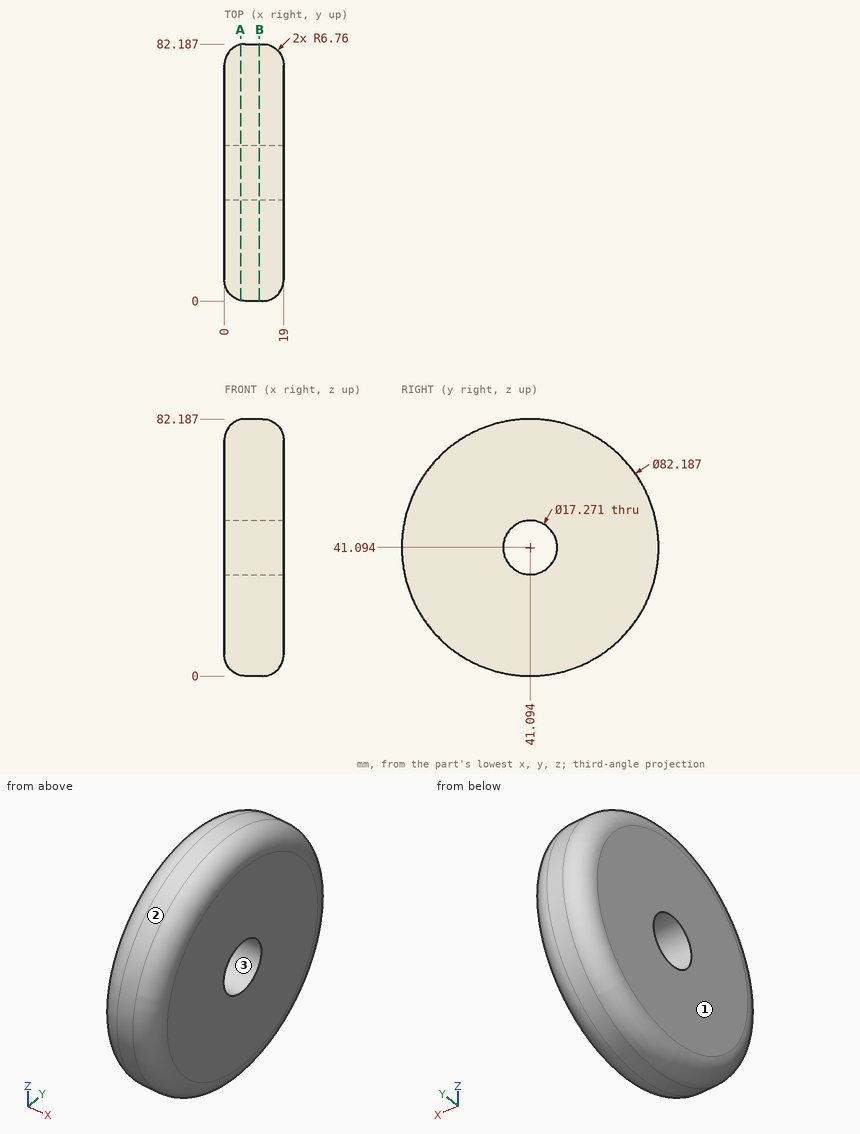
Geometry: see drawing. Coordinates: mm, zero at the bounding-box minimum. Coordinates: 2 decimals unless noted, no trailing zeros. Loops run counter-clockwise (first coordinate to the right, second up) from the corner with the lowest first, then second, coordinate; pieces in that order, holes last. Notation, with made-up numbers: M -1,58.25 L 45,58.25 A4 ccw 45,62.25 Z; hole C 2,-32.75 d3. An arc over 180 degrees is marked long. Put each result on its own line as item: value. Start each with the question number.
1) Cut plane A-A on x = 5.25. Return the cut outline in (y, z) (1 decimal), then the cut area to 3 significant figures.
2) Cut plane B-B on x = 11.25. Return the cut outline in (y, z) (1 decimal), then the cut area to 3 significant figures.
3) Ray query, L1, parallel to Z at x = 13.75, y = 39.5 (1 decimal); L2, parallel to Y at x = 7.75, z = 37.5 (1 decimal); L3, parallel to Z at x = 3.25, y = 34 (1 decimal). Return the intervals inside material, ascending. Write a range as from..to.
4) Pull-direction query (Z, two-part tool) for the marked faces 1, 2 and 3; classes: pulls with the +Z half, pulls with the -Z half, needs draft (parallel to the pull), parting line crosses it, or undercut.
5) Contact query for flat-ended pins moving along their axis: pin 1 Ø14 at (y, z) = (41.09, 41.09) entering from +X; pin 2 Ø8 at (x, z) = (2, 14.5) entering from -Y; pin 3 Ø2 at (x, y) = (2.5, 17.5) entering from -Z (1 decimal); pin 4 Ø8 at (x, y) = (10.5, 57) entering from +Z (1 decimal). Output: stop coordinate, or through.
The answers:
1. outline: C 41.1,41.1 d81.8; hole C 41.1,41.1 d17.3
1. area: 5,030 mm²
2. outline: C 41.1,41.1 d82.2; hole C 41.1,41.1 d17.3
2. area: 5,070 mm²
3. L1: z = 0.2..32.6, 49.6..82
3. L2: y = 0.2..33.2, 48.9..82
3. L3: z = 1.6..36.2, 46..80.6
4. face 1: needs draft
4. face 2: parting line crosses it
4. face 3: undercut
5. pin 1: passes through
5. pin 2: stops at y = 7.82
5. pin 3: stops at z = 8.2
5. pin 4: stops at z = 80.4
